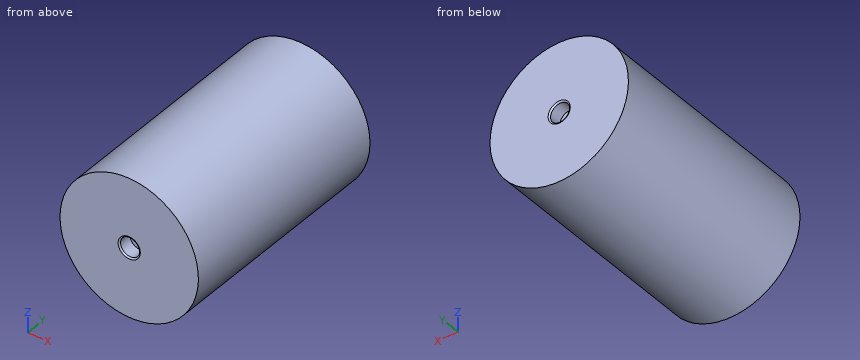
from build123d import *

# Parameters (mm, degrees)
SKETCH1_R           = 25
BOSS_EXTRUDE1_DEPTH = 82.4
SKETCH2_R           = 3.5
CUT_EXTRUDE1_DEPTH  = 5
SKETCH3_R           = 3.5
CUT_EXTRUDE2_DEPTH  = 5
FILLET1_R           = 0.5


with BuildPart() as part:
    # Sketch1 → Boss-Extrude1 (new body)
    with BuildSketch(Plane(origin=(0, 0, 0), x_dir=(1, 0, 0), z_dir=(0, 1, 0))):
        with Locations(Location((0, 0, 0), (0, 0, 270))):  # turned: the seam where the file's is
            Circle(SKETCH1_R)
    extrude(amount=BOSS_EXTRUDE1_DEPTH)

    # Sketch2 → Cut-Extrude1 (cut)
    with BuildSketch(Plane(origin=(0, 82.4, 0), x_dir=(1, 0, 0), z_dir=(0, 1, 0))):
        with Locations(Location((0, 0, 0), (0, 0, 270))):  # turned: the seam where the file's is
            Circle(SKETCH2_R)
    extrude(amount=-CUT_EXTRUDE1_DEPTH, mode=Mode.SUBTRACT)

    # Sketch3 → Cut-Extrude2 (cut)
    with BuildSketch(Plane.XZ):
        with Locations(Location((0, 0, 0), (0, 0, 90))):  # turned: the seam where the file's is
            Circle(SKETCH3_R)
    extrude(amount=-CUT_EXTRUDE2_DEPTH, mode=Mode.SUBTRACT)

    # Fillet1
    fillet1_edges = [part.edges().sort_by_distance(p)[0] for p in [
        (0, 0, -3.5),
        (0, 82.4, -3.5),
    ]]
    fillet(fillet1_edges, radius=FILLET1_R)


solid = part.part
Geometry check sheet. Reference: the model listing, model coordinates, mm. Coordinates: 2 decimals unless noted, no trailing zeros. Write each loop counter-clockwise with the first axis right and the second up, starting at its lowest first coordinate (ties: lowest second). Pieces come first, ordered by that corner, then holes. Notation, with made-up numbers: (-1.5, -30.5) -> (29.5, -30.5) arc R15 cw to (29.5, -24.5) -> close; hole circle Ø6 at (27.5, 66). An arc over 180 degrees is marked (long way). One line per question, with ' | ' between items.
1. Cross-section at B-B on z = 0. Record the cut outline in (x, y), and give its area (3 significant figures).
Answers:
outline: (-25, 0) -> (-4, 0) arc R0.5 ccw to (-3.5, 0.5) -> (-3.5, 5) -> (3.5, 5) -> (3.5, 0.5) arc R0.5 ccw to (4, 0) -> (25, 0) -> (25, 82.4) -> (4, 82.4) arc R0.5 ccw to (3.5, 81.9) -> (3.5, 77.4) -> (-3.5, 77.4) -> (-3.5, 81.9) arc R0.5 ccw to (-4, 82.4) -> (-25, 82.4) -> close | area: 4,050 mm²
2. Cross-section at C-C on y = 14.5. Record the cut outline in (x, z), and give its area (3 significant figures).
Answers:
outline: circle Ø50 at (0, 0) | area: 1,960 mm²
3. Thickness scan on probe 1 along X at (y, z) = (79.85, 0); probe 2 along Y at (x, z) = (-1, -0.5); probe 3 along Z at (x, y) = (12, 19.5). Record the ranges inside material, lowest first. Write a range as from..to.
Answers:
probe 1: x = -25..-3.5, 3.5..25 | probe 2: y = 5..77.4 | probe 3: z = -21.93..21.93
4. Depth check by flat-ended pin: pin 1 Ø1.5 at (y, z) = (10, 17.5) entering from -X; pin 2 Ø5.5 at (x, z) = (-0.5, 1.5) entering from -Y; pin 3 Ø1 at (x, y) = (16.5, 35) entering from -Z; pin 4 Ø5.5 at (x, z) = (0, 0) entering from +Y. Enter the tip coordinate at first touch or a pass-through.
Answers:
pin 1: stops at x = -18.56 | pin 2: stops at y = 0 | pin 3: stops at z = -19.21 | pin 4: stops at y = 77.4
5. Cross-section at D-D on z = 10.5. Record the cut outline in (x, y).
Answers:
outline: (-22.69, 0) -> (22.69, 0) -> (22.69, 82.4) -> (-22.69, 82.4) -> close
6. Cross-section at A-A on x = 0. Record the cut outline in (y, z), and give its area (3 significant figures).
Answers:
outline: (0, -25) -> (82.4, -25) -> (82.4, -4) arc R0.5 ccw to (81.9, -3.5) -> (77.4, -3.5) -> (77.4, 3.5) -> (81.9, 3.5) arc R0.5 ccw to (82.4, 4) -> (82.4, 25) -> (0, 25) -> (0, 4) arc R0.5 ccw to (0.5, 3.5) -> (5, 3.5) -> (5, -3.5) -> (0.5, -3.5) arc R0.5 ccw to (0, -4) -> close | area: 4,050 mm²
